```python
from build123d import *

# Parameters (mm, degrees)
F1_DEPTH = 20
F3_DEPTH = 12.7


with BuildPart() as f1:
    # F0 (on Top) → F1 (new body)
    with BuildSketch(Plane.XY):
        with BuildLine():
            ThreePointArc((-2.28661, -1.527716), (-0.798224, 2.631604), (2.75, 0))
            ThreePointArc((2.75, 0), (2.631604, -0.798224), (2.28661, -1.527716))
            Line((2.28661, -1.527716), (1.535176, -3.421364))
            ThreePointArc((1.535176, -3.421364), (3.147968, -2.037841), (3.75, 0))
            ThreePointArc((3.75, 0), (-2.037841, 3.147968), (-1.535176, -3.421364))
            Line((-1.535176, -3.421364), (-2.28661, -1.527716))
        make_face()
    extrude(amount=F1_DEPTH)

    # F2 (on Right) → F3 (cut, symmetric)
    with BuildSketch(Plane.YZ):
        with BuildLine():
            Line((-3.45, 20), (-3.45, 13))
            ThreePointArc((-3.45, 13), (-0.981115, 17.663433), (3.75, 20))
            Line((3.75, 20), (-3.45, 20))
        make_face()
    extrude(amount=F3_DEPTH, both=True, mode=Mode.SUBTRACT)


solid = f1.part
```
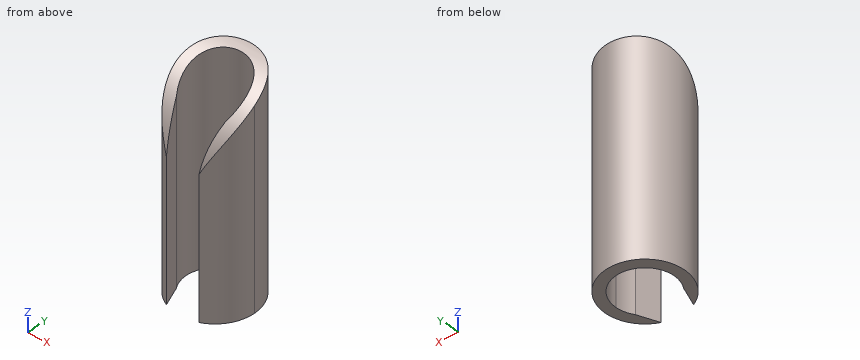
The listing builds one solid part. Answer for the finished solid, in the listing's coordinates (mm). Coordinates: 2 decimals unless noted, no trailing zeros. Loops run counter-clockwise (first coordinate to the right, second up) from the corner with the lowest first, then second, coordinate; pieces in that order, holes last. Notation, with made-up numbers: (52, 65) - (102, 65) arc R26 ccw to (102, 79) - close; hole circle Ø7 at (38.5, 47.5). An arc over 180 degrees is marked (long way). Write item = value, one per line.
1) Section D-D (x = 0) is taken. Determine the outline of the cut face in (y, z).
Responses:
outline = (2.75, 0) - (3.75, 0) - (3.75, 20) arc R8.58 ccw to (2.75, 19.79) - close
2) Section C-C (x = -1.75) is taken. Determine the outline of the cut face in (y, z), plus the area to 3 significant figures.
Responses:
outline = (-3.32, 0) - (-2.88, 0) - (-2.88, 14.91) arc R8.58 ccw to (-3.32, 13.62) - close; (2.12, 0) - (3.32, 0) - (3.32, 19.92) arc R8.58 ccw to (2.12, 19.59) - close
area = 29.9 mm^2
3) Each of these flat-tipped pins is pushed along its axis until it touches: P1, Ø4, axis at x = -2.5, z = 10.5, coming from the -Y side; P2, Ø2, axis at x = 0.5, y = 0, coming from the +Z side. Where does it stop, or does it pass through?
Responses:
P1 = -3.42
P2 = through
4) Section A-A (y = 1) is taken. Determine the outline of the cut face in (x, z).
Responses:
outline = (-3.61, 0) - (-2.56, 0) - (-2.56, 19.1) - (-3.61, 19.1) - close; (2.56, 0) - (3.61, 0) - (3.61, 19.1) - (2.56, 19.1) - close
5) Find the intervals of material crossed by line 1 along X through (y, z) = (0, 15.5); line 2 along X through (y, z) = (-2.5, 10.25); line 3 along Y through (x, z) = (0, 6), in increasing order.
Responses:
line_1 = -3.75 to -2.75, 2.75 to 3.75
line_2 = -2.8 to -1.9, 1.9 to 2.8
line_3 = 2.75 to 3.75
6) Section B-B (z = 5.25) is taken. Determine the outline of the cut face in (x, y).
Responses:
outline = (-2.29, -1.53) arc R2.75 cw (long way) to (2.75, 0) arc R2.75 cw to (2.29, -1.53) - (1.54, -3.42) arc R3.75 ccw (long way) to (-1.54, -3.42) - close
